from build123d import *

# Parameters (mm, degrees)
SKETCH1_W           = 115
SKETCH1_H           = 66
BOSS_EXTRUDE1_DEPTH = 1.75
SKETCH2_R           = 2
CUT_EXTRUDE1_DEPTH  = 1.75
SKETCH3_W           = 17.275912382
SKETCH3_H           = 11.328467136
BOSS_EXTRUDE2_DEPTH = 12
SKETCH4_W           = 29.359610659
SKETCH4_H           = 31.719707979
BOSS_EXTRUDE3_DEPTH = 34
SKETCH5_R           = 9.232777937
BOSS_EXTRUDE4_DEPTH = 34
SKETCH6_W           = 9.534793173
SKETCH6_H           = 20.013625273
BOSS_EXTRUDE5_DEPTH = 12
SKETCH7_W           = 18.314355202
SKETCH7_H           = 1.793673963
SKETCH7_W_2         = 1.604866178
SKETCH7_H_2         = 62.967396494
SKETCH7_W_3         = 15.859853989
SKETCH7_H_3         = 1.888077856
SKETCH7_H_4         = 1.416058391
SKETCH7_W_4         = 16.709489025
SKETCH7_H_5         = 2.076885642
SKETCH7_W_5         = 16.803892917
SKETCH7_H_6         = 1.982481748
BOSS_EXTRUDE6_DEPTH = 31
BOSS_EXTRUDE7_DEPTH = 31
SKETCH9_W           = 11.611678814
SKETCH9_H           = 31.719707979
CUT_EXTRUDE2_DEPTH  = 1
SKETCH11_W          = 18.503162988
SKETCH11_H          = 5.097810211
SKETCH11_H_2        = 4.814598532
BOSS_EXTRUDE8_DEPTH = 11


with BuildPart() as part:
    # Sketch1 → Boss-Extrude1 (new body)
    with BuildSketch(Plane(origin=(0, 0, 0), x_dir=(1, 0, 0), z_dir=(0, 1, 0))):
        with Locations((13.127229489, -7.155766944)):
            Rectangle(SKETCH1_W, SKETCH1_H)
    extrude(amount=BOSS_EXTRUDE1_DEPTH)

    # Sketch2 → Cut-Extrude1 (cut)
    with BuildSketch(Plane(origin=(0, 1.75, 0), x_dir=(1, 0, 0), z_dir=(0, 1, 0))):
        with Locations((65.627229489, 20.844233056)):
            Circle(SKETCH2_R)
        with Locations((65.627229489, -35.155766944)):
            Circle(SKETCH2_R)
        with Locations((-39.372770511, 20.844233056)):
            Circle(SKETCH2_R)
        with Locations((-39.372770511, -35.155766944)):
            Circle(SKETCH2_R)
    extrude(amount=-CUT_EXTRUDE1_DEPTH, mode=Mode.SUBTRACT)

    # Sketch3 → Boss-Extrude2 (add)
    with BuildSketch(Plane(origin=(0, 1.75, 0), x_dir=(1, 0, 0), z_dir=(0, 1, 0))):
        with Locations((-25.200750986, 17.672456861)):
            Rectangle(SKETCH3_W, SKETCH3_H)
    extrude(amount=BOSS_EXTRUDE2_DEPTH)

    # Sketch4 → Boss-Extrude3 (add)
    with BuildSketch(Plane(origin=(0, 1.75, 0), x_dir=(1, 0, 0), z_dir=(0, 1, 0))):
        with Locations((16.431365737, -19.711484686)):
            Rectangle(SKETCH4_W, SKETCH4_H)
    extrude(amount=BOSS_EXTRUDE3_DEPTH)

    # Sketch5 → Boss-Extrude4 (add)
    with BuildSketch(Plane(origin=(0, 1.75, 0), x_dir=(1, 0, 0), z_dir=(0, 1, 0))):
        with Locations((-14.202697476, -27.074988324)):
            Circle(SKETCH5_R)
    extrude(amount=BOSS_EXTRUDE4_DEPTH)

    # Sketch6 → Boss-Extrude5 (add)
    with BuildSketch(Plane(origin=(0, 1.75, 0), x_dir=(1, 0, 0), z_dir=(0, 1, 0))):
        with Locations((62.028445957, -0.453090556)):
            Rectangle(SKETCH6_W, SKETCH6_H)
    extrude(amount=BOSS_EXTRUDE5_DEPTH)

    # Sketch7 → Boss-Extrude6 (add)
    with BuildSketch(Plane(origin=(0, 1.75, 0), x_dir=(1, 0, 0), z_dir=(0, 1, 0))):
        with Locations((48.764699019, -27.688613628)):
            Rectangle(SKETCH7_W, SKETCH7_H)
        with Locations((38.805088329, -7.769392247)):
            Rectangle(SKETCH7_W_2, SKETCH7_H_2)
        with Locations((47.537448413, -32.833625784)):
            Rectangle(SKETCH7_W_3, SKETCH7_H_3)
        with Locations((47.537448413, -38.545061299)):
            Rectangle(SKETCH7_W_3, SKETCH7_H_4)
        with Locations((48.764699019, 11.252992151)):
            Rectangle(SKETCH7_W, SKETCH7_H_3)
        with Locations((47.962265931, 22.675863179)):
            Rectangle(SKETCH7_W_4, SKETCH7_H_5)
        with Locations((48.009467877, 18.380486057)):
            Rectangle(SKETCH7_W_5, SKETCH7_H_6)
    extrude(amount=BOSS_EXTRUDE6_DEPTH)

    # Sketch8 → Boss-Extrude7 (add)
    with BuildSketch(Plane(origin=(0, 1.75, 0), x_dir=(1, 0, 0), z_dir=(0, 1, 0))):
        Polygon((-13.541870226, 21.543016466), (-9.197015675, 21.543016466), (-9.197015675, 15.784379005), (-13.541870226, 15.784379005), (-13.541870226, 14.27391672), (-9.197015675, 14.27391672), (-9.197015675, 9.459318188), (-13.541870226, 9.459318188), (-13.541870226, 7.85445201), (-9.197015675, 7.85445201), (-9.197015675, 0), (-13.541870226, 0), (-13.541870226, -1.680341162), (-9.197015675, -1.680341162), (-9.197015675, -8.150462062), (-13.539594744, -8.150462062), (-13.539594744, -9.849732132), (-9.197015675, -9.849732132), (-9.197015675, -14.613674475), (-13.541870226, -14.613674475), (-13.541870226, -16.218540652), (-0.702940806, -16.218540652), (-0.702940806, -14.613674475), (-6.555982159, -14.613674475), (-6.555982159, 21.543016466), (-0.702940806, 21.543016466), (-0.702940806, 22.959074858), (-13.541870226, 22.959074858), align=None)
    extrude(amount=BOSS_EXTRUDE7_DEPTH)

    # Sketch9 → Cut-Extrude2 (cut)
    with BuildSketch(Plane(origin=(0, 35.75, 0), x_dir=(1, 0, 0), z_dir=(0, 1, 0))):
        with Locations((16.808981308, -19.711484686)):
            Rectangle(SKETCH9_W, SKETCH9_H)
    extrude(amount=-CUT_EXTRUDE2_DEPTH, mode=Mode.SUBTRACT)

    # Sketch11 → Boss-Extrude8 (add)
    with BuildSketch(Plane(origin=(0, 1.75, 0), x_dir=(1, 0, 0), z_dir=(0, 1, 0))):
        with Locations((-29.496128108, 5.494354691)):
            Rectangle(SKETCH11_W, SKETCH11_H)
        with Locations((-29.496128108, -14.755280314)):
            Rectangle(SKETCH11_W, SKETCH11_H_2)
    extrude(amount=BOSS_EXTRUDE8_DEPTH)


solid = part.part
Work out the finished part from the listing and answer in its coordinate system (mm). A direction names the side the tool comes from. Give positions to 0.01 mm unless a question says otherwise; leave off trailing zeros. Loops run counter-clockwise (first coordinate to the right, second up) from the corner with the lowest first, then second, coordinate; pieces in that order, holes last. Notation, with made-up numbers: M -19,29.5 L -10,29.5 A10 ccw -10,41.5 Z; hole C 64,-14 d3. An arc over 180 degrees is marked long. Use CSV: the item, a comma, the result in double quotes.
1) Find section B-B on x = -25. Write down the section's boundary in (y, z), plus the area to 3 significant figures.
Answer:
outline,"M 0,-25.84 L 1.75,-25.84 L 1.75,-23.34 L 13.75,-23.34 L 13.75,-12.01 L 1.75,-12.01 L 1.75,-8.04 L 12.75,-8.04 L 12.75,-2.95 L 1.75,-2.95 L 1.75,12.35 L 12.75,12.35 L 12.75,17.16 L 1.75,17.16 L 1.75,40.16 L 0,40.16 Z"
area,"360 mm^2"
2) Find section D-D on x = 26. Write down the section's boundary in (y, z), plus the area to 3 significant figures.
Answer:
outline,"M 0,-25.84 L 1.75,-25.84 L 1.75,3.85 L 35.75,3.85 L 35.75,35.57 L 1.75,35.57 L 1.75,40.16 L 0,40.16 Z"
area,"1,190 mm^2"
3) Consider L1, parallel to X at y = 6, z = 10; L2, parallel to Z at x = -30, y = 3.5; L3, parallel to X at y = 7, z = -7. Determine where each line is inside the solid, lowest interval first.
Answer:
L1,"-9.2 to -6.56, 1.75 to 31.11, 38 to 39.61, 57.26 to 66.8"
L2,"-23.34 to -12.01, -8.04 to -2.95, 12.35 to 17.16"
L3,"-38.75 to -20.24, -9.2 to -6.56, 38 to 39.61, 57.26 to 66.8"
4) Which of the six approach directions +Z, -Z, +X, -X, +Y, -Y give full straight-line access (tool end or side, diameter ignored) to faces 1 (the flat face through (-30, 7, -8.043)), 2 (the flat face through (-25, 13.75, -18)), 3 (the flat face through (47, 17, 37.837))?
Answer:
face 1,"-X, +Y"
face 2,"-Z, -X, +Y"
face 3,"+X, +Y"
5) Given P1, Ø3, axis at y = 21.5, z = -13, coming from the -X side; P2, Ø1.3, axis at x = -11.5, y = 17, coming from the +Z side; P3, Ø0.6, axis at y = 22, z = -23, coming from the +X side, each flat-ended and moving along its own axis, determine where each tip first touches the part or whether it passes through.
Answer:
P1,"x = -13.54"
P2,"z = 36.08"
P3,"x = 56.32"
6) Find section C-C on y = 25. Give the number of separate pieces and of enclosed holes in the cut face, plus the area to 3 significant figures.
Answer:
separate pieces,"4"
enclosed holes,"0"
area,"1,650 mm^2"
7) Find section A-A on z = 7. Write down the section's boundary in (x, y).
Answer:
outline,"M -44.37,0 L 70.63,0 L 70.63,1.75 L 66.8,1.75 L 66.8,13.75 L 57.26,13.75 L 57.26,1.75 L 39.61,1.75 L 39.61,32.75 L 38,32.75 L 38,1.75 L 31.11,1.75 L 31.11,35.75 L 22.61,35.75 L 22.61,34.75 L 11,34.75 L 11,35.75 L 1.75,35.75 L 1.75,1.75 L -6.56,1.75 L -6.56,32.75 L -9.2,32.75 L -9.2,1.75 L -44.37,1.75 Z"
